```python
from build123d import *

# Parameters (mm, degrees)
F0_R     = 1.84
F1_DEPTH = 1.53
F2_R     = 1
F3_R     = 0.5


with BuildPart() as f1:
    # F0 (on Top) → F1 (new body)
    with BuildSketch(Plane.XY):
        with BuildLine():
            Line((-9.765, 28.690863), (-9.765, 25.180746))
            Line((-9.765, 25.180746), (-9.765, 23.540863))
            Line((-9.765, 23.540863), (-6.612455, 21.610863))
            Line((-6.612455, 21.610863), (-6.612455, 14.620863))
            Line((-6.612455, 14.620863), (-9.765, 12.690863))
            Line((-9.765, 12.690863), (-9.765, -25.956517))
            Line((-9.765, -25.956517), (-3.835, -25.956517))
            Line((-3.835, -25.956517), (-3.618682, 7.628455))
            ThreePointArc((-3.618682, 7.628455), (-3.659924, 8.200425), (-3.611318, 8.771817))
            ThreePointArc((-3.611318, 8.771817), (0, 11.836852), (3.611318, 8.771817))
            Line((3.611318, 8.771817), (3.835, -25.956517))
            Line((3.835, -25.956517), (9.765, -25.956517))
            Line((9.765, -25.956517), (9.765, 12.690863))
            Line((9.765, 12.690863), (6.612455, 14.620863))
            Line((6.612455, 14.620863), (6.612455, 21.610863))
            Line((6.612455, 21.610863), (9.765, 23.540863))
            Line((9.765, 23.540863), (9.765, 25.180746))
            Line((9.765, 25.180746), (9.765, 28.690863))
            Line((9.765, 28.690863), (-9.765, 28.690863))
        make_face()
        with Locations((-6.8, 26.120863)):
            Circle(F0_R, mode=Mode.SUBTRACT)
        with Locations((6.8, 26.120863)):
            Circle(F0_R, mode=Mode.SUBTRACT)
        Polygon((-3.835, -25.956517), (-9.765, -25.956517), (-6.8, -31.106517), align=None)
        with BuildLine():
            ThreePointArc((-3.611318, 8.771817), (-3.659924, 8.200425), (-3.618682, 7.628455))
            Line((-3.618682, 7.628455), (-3.611318, 8.771817))
        make_face()
        Polygon((6.8, -31.106517), (9.765, -25.956517), (3.835, -25.956517), align=None)
    extrude(amount=F1_DEPTH)

    # F2
    f2_edges = [f1.edges().sort_by_distance(p)[0] for p in [
        (6.612455, 21.610863, 0.765),
        (6.612455, 14.620863, 0.765),
        (-6.612455, 21.610863, 0.765),
        (-6.612455, 14.620863, 0.765),
    ]]
    fillet(f2_edges, radius=F2_R)

    # F3
    f3_edges = [f1.edges().sort_by_distance(p)[0] for p in [
        (-6.8, -31.106517, 0.765),
        (6.8, -31.106517, 0.765),
    ]]
    fillet(f3_edges, radius=F3_R)


solid = f1.part
```
Geometry check sheet. Reference: the model listing, model coordinates, mm. A direction names the side the tool comes from. Coordinates: 2 decimals unless noted, no trailing zeros. Loops run counter-clockwise (first coordinate to the right, second up) from the corner with the lowest first, then second, coordinate; pieces in that order, holes last. Notation, with made-up numbers: (-34, 60.25) -> (-11, 60.25) arc R9 cw to (-11, 72.25) -> close; hole circle Ø6 at (63, 37). An arc over 180 degrees is marked (long way). Put each result on its own line as item: value.
1) Thickness scan on line 1 (Y direction, x = 6.8, z = 0.9); line 2 (X direction, y = 24.5, z = 0.2) (3 decimals); line 3 (X direction, y = -25, z = 1.2) (3 decimals). Record the ranges inside material, lowest first.
Result set:
line 1: y = -30.6 to 14.6, 21.63 to 24.28, 27.96 to 28.69
line 2: x = -9.765 to -7.671, -5.929 to 5.929, 7.671 to 9.765
line 3: x = -9.765 to -3.829, 3.829 to 9.765
2) Cross-section at C-C on y = -1. Record the boundary of the cut face in (x, z) (3 decimals).
Result set:
outline: (-9.765, 0) -> (-3.674, 0) -> (-3.674, 1.53) -> (-9.765, 1.53) -> close; (3.674, 0) -> (9.765, 0) -> (9.765, 1.53) -> (3.674, 1.53) -> close
3) Release check for a two-part mould opening along X. For faces 1 (the cylindrical face through (-0.072, 11.836, 0.754)), 2 (the flat face through (-8.41, 13.52, 0.75)), 3 (the flat face through (8.41, 22.71, 0.75)) record: released by +X, released by -X, zero draft, split by the parting line, or undercut.
Result set:
face 1: undercut
face 2: released by -X
face 3: released by +X
4) Cross-section at A-A on y = -15.5. Record the boundary of the cut face in (x, z) (3 decimals), plus the area to 3 significant figures.
Result set:
outline: (-9.765, 0) -> (-3.768, 0) -> (-3.768, 1.53) -> (-9.765, 1.53) -> close; (3.768, 0) -> (9.765, 0) -> (9.765, 1.53) -> (3.768, 1.53) -> close
area: 18.4 mm^2
5) Gauge pin test, flat ends, axial feed: pin 1 Ø0.8 at (y, z) = (19.5, 0.5) entering from +X; pin 2 Ø3 at (x, y) = (-6.8, 26.12) entering from -Z. Record the tip position at first contact, or that the pin passes through.
Result set:
pin 1: stops at x = 6.61
pin 2: passes through
6) Tool access check on faces 4 (the flat face through (-8.446, 22.734, 0.754)), 5 (the flat face through (-5.12, -28.19, 0.75)), 6 (the flat face through (8.446, 13.498, 0.754)), 7 (the flat face through (-9.765, -6, 1)). Record the directions out of +Z, -Z, +X, -X, +Y, -Y that give a thin tool (end or side, any length) a straight path to the whole face; none if there is none.
Result set:
face 4: +Z, -Z, -X
face 5: +Z, -Z, -Y
face 6: +Z, -Z, +X
face 7: +Z, -Z, -X, +Y, -Y
7) Cross-section at D-D on x = 1. Record the boundary of the cut face in (y, z).
Result set:
outline: (11.7, 0) -> (28.69, 0) -> (28.69, 1.53) -> (11.7, 1.53) -> close
8) Cross-section at B-B on z = 0.6. Record the boundary of the cut face in (x, y) (3 decimals), plus the area to 3 significant figures.
Result set:
outline: (-9.765, -25.957) -> (-7.233, -30.354) arc R0.5 ccw to (-6.367, -30.354) -> (-3.835, -25.957) -> (-3.619, 7.628) -> (-3.611, 8.772) arc R3.66 cw to (3.611, 8.772) -> (3.835, -25.957) -> (6.367, -30.354) arc R0.5 ccw to (7.233, -30.354) -> (9.765, -25.957) -> (9.765, 12.691) -> (7.09, 14.328) arc R1 cw to (6.612, 15.181) -> (6.612, 21.051) arc R1 cw to (7.09, 21.903) -> (9.765, 23.541) -> (9.765, 28.691) -> (-9.765, 28.691) -> (-9.765, 23.541) -> (-7.09, 21.903) arc R1 cw to (-6.612, 21.051) -> (-6.612, 15.181) arc R1 cw to (-7.09, 14.328) -> (-9.765, 12.691) -> close; hole circle Ø3.68 at (-6.8, 26.121); hole circle Ø3.68 at (6.8, 26.121)
area: 745 mm^2
